```python
from build123d import *

# Parameters (mm, degrees)
SKETCH1_W                                   = 499.3132
SKETCH1_H                                   = 797.0266
SIDEPANEL_DEPTH                             = 3.0734
SKETCH2_R                                   = 2.8956
TOPBOTTOMHOLEMASTER_DEPTH                   = 4.0734
LPATTERN1_COUNT                             = 4
LPATTERN1_PITCH                             = 127.067733333
SKETCH3_R                                   = 2.8956
REARHOLESMASTER_DEPTH                       = 4.0734
LPATTERN2_COUNT                             = 4
LPATTERN2_PITCH                             = 211.7344
SKETCH4_W                                   = 19.05
SKETCH4_H                                   = 19.05
SKETCH4_W_2                                 = 22.86
CORNERCUTS_DEPTH                            = 4.0734
F_8_CLEARANCE_HOLE4_BRAIN_MOUNT_D           = 7.8232
F_8_CLEARANCE_HOLE3_PUMP_MOUNTS_D           = 4.4958
SKETCH17_W                                  = 25.4
SKETCH17_H                                  = 50.8
CABLE_PASS_THROUGH_DEPTH                    = 4.0734
F_8_CLEARANCE_HOLE1_PASS_THROUGH_MOUNTING_D = 7.8232
CUT_EXTRUDE1_DEPTH                          = 2.54
F_8_CLEARANCE_HOLE_HX_MOUNT_D               = 7.8232
SKETCH42_R                                  = 7.578725
SKETCH42_R_2                                = 7.5819
COOLANT_HOSE_PASS_THROUGH_DEPTH             = 4.0734
SKETCH43_R                                  = 7.5819
AIR_FLUSH_IN_OUT_DEPTH                      = 4.0734
F_8_CLEARANCE_HOLE2_AIR_FLUSH_OUT_MOUNT_D   = 7.8232
F_8_CLEARANCE_HOLE4_PANEL_MOUNTS_D          = 7.8232
FILLET1_R                                   = 3.81
SKETCH50_OUTSIDE_W                          = 689.418
SKETCH50_OUTSIDE_H                          = 987.13
SKETCH50_OUTSIDE_R                          = 8.1915
SENSOR_MOUNTING_DEPTH                       = 4.0734
F_8_CLEARANCE_HOLE1_D                       = 4.4958
F_12_CLEARANCE_HOLE1_D                      = 5.7912
FILLET2_R                                   = 0.127
F_4_CLEARANCE_HOLE_COMPRESSOR_DRIVER_D      = 5.7912
F_1_4_CLEARANCE_HOLE_BALL_VALVE_U_BOLT_D    = 6.5278
AERATION_PUMP_8_CLEARANCE_HOLE1_D           = 4.3053
NUTRIENT_HOLES_R                            = 3.0226
NUTRIENT_HOSES_DEPTH                        = 4.0734
LPATTERN3_COUNT                             = 3
LPATTERN3_PITCH                             = 12.7
LPATTERN3_COUNT_DIR2                        = 3
LPATTERN3_PITCH_DIR2                        = 12.7
SKETCH61_W                                  = 508.2032
SKETCH61_H                                  = 809.7266
SKETCH61_W_2                                = 457.4032
SKETCH61_H_2                                = 758.9266
CUT_EXTRUDE2_DEPTH                          = 4.0734


with BuildPart() as part:
    # Sketch1 → SidePanel (new body)
    with BuildSketch(Plane(origin=(0, 0, 0), x_dir=(0, 0, -1), z_dir=(1, 0, 0))):
        Rectangle(SKETCH1_W, SKETCH1_H)
    extrude(amount=SIDEPANEL_DEPTH)

    # Sketch2 → TopBottomHoleMaster (cut, through all)
    with BuildSketch(Plane(origin=(3.0734, 0, 0), x_dir=(0, 0, -1), z_dir=(1, 0, 0))):
        with Locations((192.5066, 388.9883)):
            Circle(SKETCH2_R)
        with Locations((192.5066, -388.9883)):
            Circle(SKETCH2_R)
    topbottomholemaster = extrude(amount=-TOPBOTTOMHOLEMASTER_DEPTH, mode=Mode.SUBTRACT)

    # LPattern1: TopBottomHoleMaster ×4
    with Locations(*[(0, 0, i * LPATTERN1_PITCH) for i in range(1, LPATTERN1_COUNT)]):
        add(topbottomholemaster, mode=Mode.SUBTRACT)

    # Sketch3 → RearHolesMaster (cut, through all)
    with BuildSketch(Plane(origin=(3.0734, 0, 0), x_dir=(0, 0, -1), z_dir=(1, 0, 0))):
        with Locations((-236.3216, 315.8617)):
            Circle(SKETCH3_R)
        with Locations((240.1316, 315.8617)):
            Circle(SKETCH3_R)
    rearholesmaster = extrude(amount=-REARHOLESMASTER_DEPTH, mode=Mode.SUBTRACT)

    # LPattern2: RearHolesMaster ×4
    with Locations(*[(0, -i * LPATTERN2_PITCH, 0) for i in range(1, LPATTERN2_COUNT)]):
        add(rearholesmaster, mode=Mode.SUBTRACT)

    # Sketch4 → CornerCuts (cut, through all)
    with BuildSketch(Plane.ZY):
        with Locations((-240.1316, 388.9883)):
            Rectangle(SKETCH4_W, SKETCH4_H)
        with Locations((238.2266, 388.9883)):
            Rectangle(SKETCH4_W_2, SKETCH4_H)
        with Locations((-240.1316, -388.9883)):
            Rectangle(SKETCH4_W, SKETCH4_H)
    extrude(amount=-CORNERCUTS_DEPTH, mode=Mode.SUBTRACT)

    # #8 Clearance Hole4 Brain Mount (through all)
    with Locations(Plane.ZY):
        with Locations((-23.3934, 344.4367), (52.8066, 344.4367), (52.8066, -61.9633), (-23.3934, -61.9633), (-146.4564, 141.8717), (-146.4564, 247.2817), (61.5696, 197.49262), (61.5696, 113.41862)):
            Hole(F_8_CLEARANCE_HOLE4_BRAIN_MOUNT_D / 2)

    # #8 Clearance Hole3 Pump Mounts (through all)
    with Locations(Plane.ZY):
        with Locations((46.4566, -138.1633), (8.3566, -100.0633), (8.3566, -176.2633), (-29.7434, -138.1633)):
            Hole(F_8_CLEARANCE_HOLE3_PUMP_MOUNTS_D / 2)

    # Sketch17 → Cable Pass Through (cut, through all)
    with BuildSketch(Plane.ZY):
        with Locations((-186.1566, 322.3133)):
            Rectangle(SKETCH17_W, SKETCH17_H)
        with Locations((-186.1566, -322.3133)):
            Rectangle(SKETCH17_W, SKETCH17_H)
    extrude(amount=-CABLE_PASS_THROUGH_DEPTH, mode=Mode.SUBTRACT)

    # #8 Clearance Hole1 Pass through Mounting holes (through all)
    with Locations(Plane(origin=(3.0734, 0, 0), x_dir=(0, 0, -1), z_dir=(1, 0, 0))):
        with Locations((154.4066, -348.9833), (203.9366, -348.9833), (203.9366, -295.6433), (154.4066, -295.6433), (154.4066, 348.9833), (203.9366, 348.9833), (203.9366, 295.6433), (154.4066, 295.6433)):
            Hole(F_8_CLEARANCE_HOLE1_PASS_THROUGH_MOUNTING_D / 2)

    # Sketch39 → Cut-Extrude1 (cut)
    with BuildSketch(Plane.ZY):
        Polygon((-230.2256, 398.5133), (-230.6066, 398.5133), (-230.6066, 379.4633), (-249.6566, 379.4633), (-249.6566, 379.0823), (-230.2256, 379.0823), align=None)
        Polygon((-249.6566, -379.0823), (-249.6566, -379.4633), (-230.6066, -379.4633), (-230.6066, -398.5133), (-230.2256, -398.5133), (-230.2256, -379.0823), align=None)
        Polygon((226.7966, 398.5133), (226.4156, 398.5133), (226.4156, 379.0823), (249.6566, 379.0823), (249.6566, 379.4633), (226.7966, 379.4633), align=None)
    extrude(amount=-CUT_EXTRUDE1_DEPTH, mode=Mode.SUBTRACT)

    # #8 Clearance Hole -hx mount (through all)
    with Locations(Plane(origin=(3.0734, 0, 0), x_dir=(0, 0, -1), z_dir=(1, 0, 0))):
        with Locations((205.2066, 246.1133), (205.2066, 141.1133), (100.2066, 141.1133), (100.2066, 246.1133)):
            Hole(F_8_CLEARANCE_HOLE_HX_MOUNT_D / 2)

    # Sketch42 → Coolant hose pass through (cut, through all)
    with BuildSketch(Plane(origin=(3.0734, 0, 0), x_dir=(0, 0, -1), z_dir=(1, 0, 0))):
        with Locations((197.8406, 118.5073)):
            Circle(SKETCH42_R)
        with Locations((107.5726, 118.5073)):
            Circle(SKETCH42_R_2)
    extrude(amount=-COOLANT_HOSE_PASS_THROUGH_DEPTH, mode=Mode.SUBTRACT)

    # Sketch43 → Air flush in/out (cut, through all)
    with BuildSketch(Plane(origin=(3.0734, 0, 0), x_dir=(0, 0, -1), z_dir=(1, 0, 0))):
        with Locations((-198.8566, 347.7133)):
            Circle(SKETCH43_R)
        with Locations((107.5726, 80.4073)):
            Circle(SKETCH43_R)
    extrude(amount=-AIR_FLUSH_IN_OUT_DEPTH, mode=Mode.SUBTRACT)

    # #8 Clearance Hole2 Air Flush Out mount (through all)
    with Locations(Plane(origin=(3.0734, 0, 0), x_dir=(0, 0, -1), z_dir=(1, 0, 0))):
        with Locations((225.5266, -160.7693), (225.5266, -208.0133), (128.067808498, -181.154848387)):
            Hole(F_8_CLEARANCE_HOLE2_AIR_FLUSH_OUT_MOUNT_D / 2)

    # #8 Clearance Hole4 Panel Mounts (through all)
    with Locations(Plane(origin=(3.0734, 0, 0), x_dir=(0, 0, -1), z_dir=(1, 0, 0))):
        with Locations((-217.7034, 230.1367), (-217.7034, -49.2633)):
            Hole(F_8_CLEARANCE_HOLE4_PANEL_MOUNTS_D / 2)

    # Fillet1
    fillet1_edges = [part.edges().sort_by_distance(p)[0] for p in [
        (1.5367, 296.9133, -198.8566),
        (1.5367, 347.7133, -198.8566),
        (1.5367, 347.7133, -173.4566),
        (1.5367, 296.9133, -173.4566),
        (1.5367, -347.7133, -173.4566),
        (1.5367, -347.7133, -198.8566),
        (1.5367, -296.9133, -198.8566),
        (1.5367, -296.9133, -173.4566),
    ]]
    fillet(fillet1_edges, radius=FILLET1_R)

    # Sketch50 outside → Sensor Mounting (cut, through all)
    with BuildSketch(Plane(origin=(3.0734, 0, 0), x_dir=(0, 0, -1), z_dir=(1, 0, 0))):
        Rectangle(SKETCH50_OUTSIDE_W, SKETCH50_OUTSIDE_H)
        Polygon((230.6066, -379.4633), (249.6566, -379.4633), (249.6566, 379.4633), (230.6066, 379.4633), (230.6066, 398.5133), (-226.7966, 398.5133), (-226.7966, 379.4633), (-249.6566, 379.4633), (-249.6566, -398.5133), (230.6066, -398.5133), align=None, mode=Mode.SUBTRACT)
        with Locations((127, -4.8133)):
            Circle(SKETCH50_OUTSIDE_R)
        with Locations((127, 38.3667)):
            Circle(SKETCH50_OUTSIDE_R)
        Polygon((-8.625, 3.8117), (8.625, 3.8117), (8.625, -2.6883), (12.125, -2.6883), (12.125, -6.9383), (8.625, -6.9383), (8.625, -13.4383), (-8.625, -13.4383), (-8.625, -6.9383), (-12.125, -6.9383), (-12.125, -2.6883), (-8.625, -2.6883), align=None)
    extrude(amount=-SENSOR_MOUNTING_DEPTH, mode=Mode.SUBTRACT)

    # #8 Clearance Hole1 (through all)
    with Locations(Plane(origin=(3.0734, 0, 0), x_dir=(0, 0, -1), z_dir=(1, 0, 0))):
        with Locations((-13.97, 9.1567), (13.97, 9.1567), (13.97, -18.7833), (-13.97, -18.7833)):
            Hole(F_8_CLEARANCE_HOLE1_D / 2)

    # #12 Clearance Hole1 (through all)
    with Locations(Plane(origin=(3.0734, 0, 0), x_dir=(0, 0, -1), z_dir=(1, 0, 0))):
        with Locations((98, 38.3667), (156, 38.3667)):
            Hole(F_12_CLEARANCE_HOLE1_D / 2)

    # Fillet2
    fillet2_edges = [part.edges().sort_by_distance(p)[0] for p in [
        (1.5367, -2.6883, 8.625),
        (1.5367, 3.8117, 8.625),
        (1.5367, 3.8117, -8.625),
        (1.5367, -2.6883, -8.625),
        (1.5367, -2.6883, -12.125),
        (1.5367, -6.9383, -12.125),
        (1.5367, -6.9383, -8.625),
        (1.5367, -13.4383, -8.625),
        (1.5367, -13.4383, 8.625),
        (1.5367, -6.9383, 8.625),
        (1.5367, -6.9383, 12.125),
        (1.5367, -2.6883, 12.125),
    ]]
    fillet(fillet2_edges, radius=FILLET2_R)

    # #4 Clearance Hole compressor driver (through all)
    with Locations(Plane.ZY):
        with Locations((-17.0434, -227.3133), (-62.0434, -227.3133), (-62.0434, -322.3133), (-17.0434, -322.3133)):
            Hole(F_4_CLEARANCE_HOLE_COMPRESSOR_DRIVER_D / 2)

    # 1/4 Clearance Hole ball valve u bolt (through all)
    with Locations(Plane(origin=(3.0734, 0, 0), x_dir=(0, 0, -1), z_dir=(1, 0, 0))):
        with Locations((220.1418, -99.7331), (185.2168, -99.7331)):
            Hole(F_1_4_CLEARANCE_HOLE_BALL_VALVE_U_BOLT_D / 2)

    # Aeration Pump #8 Clearance Hole1 (through all)
    with Locations(Plane(origin=(3.0734, 0, 0), x_dir=(0, 0, -1), z_dir=(1, 0, 0))):
        with Locations((-31.37535, -291.753925)):
            Hole(AERATION_PUMP_8_CLEARANCE_HOLE1_D / 2)

    # Nutrient Holes → Nutrient Hoses (cut, through all)
    with BuildSketch(Plane(origin=(3.0734, 0, 0), x_dir=(0, 0, -1), z_dir=(1, 0, 0))):
        with Locations((87.4434, -214.3633)):
            Circle(NUTRIENT_HOLES_R)
    nutrient_hoses = extrude(amount=-NUTRIENT_HOSES_DEPTH, mode=Mode.SUBTRACT)

    # LPattern3: Nutrient Hoses 3 × 3, 4 skipped
    with Locations(*[(0, i * LPATTERN3_PITCH, j * LPATTERN3_PITCH_DIR2) for i in range(LPATTERN3_COUNT) for j in range(LPATTERN3_COUNT_DIR2) if (i, j) not in ((0, 0), (0, 2), (1, 2), (2, 1), (2, 2))]):
        add(nutrient_hoses, mode=Mode.SUBTRACT)

    # Sketch61 → Cut-Extrude2 (cut, through all)
    with BuildSketch(Plane(origin=(3.0734, 0, 0), x_dir=(0, 0, -1), z_dir=(1, 0, 0))):
        with Locations((1.905, 0)):
            Rectangle(SKETCH61_W, SKETCH61_H)
        with Locations((1.905, 0)):
            Rectangle(SKETCH61_W_2, SKETCH61_H_2, mode=Mode.SUBTRACT)
    extrude(amount=-CUT_EXTRUDE2_DEPTH, mode=Mode.SUBTRACT)


solid = part.part
```
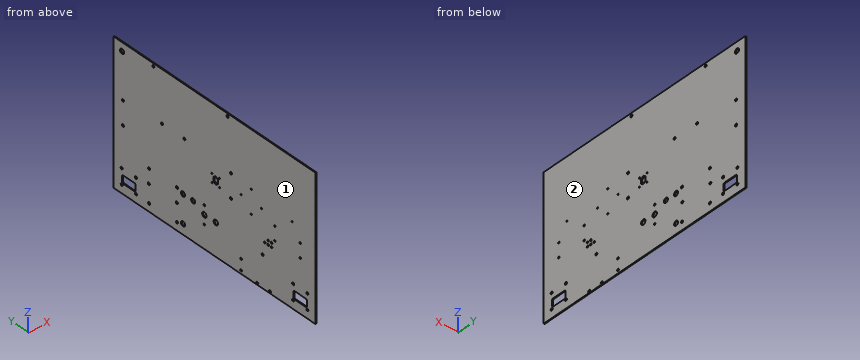
Source: CAD feature listing. Evaluate the final solid. Frame: model axes, mm. Face numbers are marked on the shaded views. Give positions to 0.01 mm unless a question says otherwise; leave off trailing zeros.
1. Pull-direction query (X, two-part tool) for the marked faces 1 and 2; classes: +X half, -X half, draft (parallel to the pull), parting line (faces both ways), or undercut.
2. Section query A-A (x = 0.8). Count the separate pieces of the cut face and the enclosed holes in it, then the cut area to 3 significant figures.
3. Material intervals for line 1 along Y through (x, z) = (1.9, -13.97); line 2 along Z through (x, y) = (2.3, -100.5); line 3 along Z through (x, y) = (2.8, -305.5), sorted ascending.
Output values:
1. face 1: -X half
1. face 2: +X half
2. separate pieces: 1
2. enclosed holes: 56
2. area: 341,000 mm2
3. line 1: y = -379.46 to -21.03, -16.54 to 6.91, 11.4 to 379.46
3. line 2: z = -230.61 to -223.31, -216.97 to -188.39, -182.04 to 6.15, 10.56 to 226.8
3. line 3: z = -230.61 to -198.86, -173.46 to 226.8
